Here's how the part is built. I have some questions about the finished solid (model axes, mm). A direction names the side the tool comes from. Coordinates: 2 decimals unless noted, no trailing zeros. Order: outer loops, then holes, each group sorted by start corner. A loop starts at its lowest first (then second) coordinate and runs counter-clockwise, first axis right, second up. Notation, with made-up numbers: (32.25, 6) - (62.25, 6) arc R27 cw to (62.25, 37) - close; hole circle Ø10 at (-35, 65.5). An arc over 180 degrees is marked (long way). Answer in a Markdown table with one row per item. Add a question column.
Item 1: I want a section at D-D (x = 4). Please give me the cut outline in (y, z), plus the area to 3 significant figures.
Item 2: I want a section at A-A (x = -24). Please give me the cut outline in (y, z), plus the area to 3 significant figures.
Item 3: Will these pins go through, and if not, where does the flat tip stop? pin 1 Ø1.5 at (x, z) = (-45.5, 5) entering from -Y; pin 2 Ø1.9 at (y, z) = (40, 4) entering from +X; pin 3 Ø3 at (y, z) = (41.5, 4) entering from -X.
Item 4: If I drill on line 1 along Y through (x, z) = (-56, 3.75); line 2 along Y through (x, z) = (-17, 4.75); line 3 along X through (y, z) = (41, 4), over which ranges is the centre line in solid material (lowest first)? Write a range as from..to.
Item 5: I want a section at C-C (z = 5.25). Please give me the cut outline in (x, y), plus the area to 3 significant figures.
Item 6: Thinking about a two-plate mould opening in Y: for faces 6 (the flat face through (-13, 38.1, 3)), 7 (the flat face through (6.35, 41, 3)), 8 (the flat face through (-43, 69.83, 3)), which applies, +Y half, -Y half, draft (parallel to the pull), parting line (faces both ways), or undercut?
Item 7: I want a section at B-B (y = 67.5). Please give me the cut outline in (x, z) (3 decimals), plus the area to 3 significant figures.
Item 8: On a 3-axis mill with a long thin cutter (end or side, diameter ignored), from which of +Z, -Z, +X, -X, +Y, -Y can I reach the whole of each face in a straight line? I mean faces 1 (the flat face through (-63.45, 59, 3)), 2 (the flat face through (27, 44.45, 3)), 3 (the cylindrical face through (-66.44, 71.28, 3.22)), 4 (the flat face through (-16, 74.13, 3)), 5 (the flat face through (-19.05, 41, 3)). Say none if no direction works.
```python
from build123d import *

# Parameters (mm, degrees)
BOSS_EXTRUDE1_DEPTH = 6.35
SKETCH3_R           = 1.778
SKETCH3_W           = 41
SKETCH3_H           = 21
CUT_EXTRUDE1_DEPTH  = 102.778507746
FILLET1_R           = 10


with BuildPart() as part:
    # Sketch1 → Boss-Extrude1 (new body)
    with BuildSketch(Plane.XY):
        Polygon((19.05, 38.1), (19.05, 44.45), (35.872396717, 44.45), (35.872396717, 74.129883576), (-49.45, 74.129883576), (-69.45, 74.129883576), (-69.45, 44.45), (-44.45, 44.45), (-19.05, 44.45), (-19.05, 38.1), (-6.35, 38.1), (-6.35, 44.45), (6.35, 44.45), (6.35, 38.1), align=None)
    extrude(amount=BOSS_EXTRUDE1_DEPTH)

    # Sketch3 → Cut-Extrude1 (cut, through all)
    with BuildSketch(Plane.XY.offset(6.35)):
        with Locations((-67.4705, 64.289941788)):
            Circle(SKETCH3_R)
        with Locations((-67.4705, 54.289941788)):
            Circle(SKETCH3_R)
        with Locations((-18.4705, 54.289941788)):
            Circle(SKETCH3_R)
        with Locations((-18.4705, 64.289941788)):
            Circle(SKETCH3_R)
        with Locations((-42.95, 59.329883576)):
            Rectangle(SKETCH3_W, SKETCH3_H)
    extrude(amount=-CUT_EXTRUDE1_DEPTH, mode=Mode.SUBTRACT)

    # Fillet1
    fillet1_edges = [part.edges().sort_by_distance(p)[0] for p in [
        (-69.45, 74.129883576, 3.175),
        (35.872396717, 74.129883576, 3.175),
    ]]
    fillet(fillet1_edges, radius=FILLET1_R)


solid = part.part
```
Values follow:
| question | item | result |
|---|---|---|
| 1 | outline | (44.45, 0) - (74.13, 0) - (74.13, 6.35) - (44.45, 6.35) - close |
| 1 | area | 188 mm^2 |
| 2 | outline | (44.45, 0) - (48.83, 0) - (48.83, 6.35) - (44.45, 6.35) - close; (69.83, 0) - (74.13, 0) - (74.13, 6.35) - (69.83, 6.35) - close |
| 2 | area | 55.1 mm^2 |
| 3 | pin 1 | stops at y = 44.45 |
| 3 | pin 2 | stops at x = 19.05 |
| 3 | pin 3 | stops at x = -19.05 |
| 4 | line 1 | y = 44.45..48.83, 69.83..74.13 |
| 4 | line 2 | y = 38.1..53.29, 55.29..63.29, 65.29..74.13 |
| 4 | line 3 | x = -19.05..-6.35, 6.35..19.05 |
| 5 | outline | (-69.45, 44.45) - (-19.05, 44.45) - (-19.05, 38.1) - (-6.35, 38.1) - (-6.35, 44.45) - (6.35, 44.45) - (6.35, 38.1) - (19.05, 38.1) - (19.05, 44.45) - (35.87, 44.45) - (35.87, 64.13) arc R10 ccw to (25.87, 74.13) - (-59.45, 74.13) arc R10 ccw to (-69.45, 64.13) - close; hole circle Ø3.56 at (-67.47, 54.29); hole circle Ø3.56 at (-67.47, 64.29); hole (-63.45, 48.83) - (-22.45, 48.83) - (-22.45, 69.83) - (-63.45, 69.83) - close; hole circle Ø3.56 at (-18.47, 54.29); hole circle Ø3.56 at (-18.47, 64.29) |
| 5 | area | 2,340 mm^2 |
| 6 | face 6 | -Y half |
| 6 | face 7 | draft |
| 6 | face 8 | undercut |
| 7 | outline | (-68.865, 0) - (-63.45, 0) - (-63.45, 6.35) - (-68.865, 6.35) - close; (-22.45, 0) - (35.287, 0) - (35.287, 6.35) - (-22.45, 6.35) - close |
| 7 | area | 401 mm^2 |
| 8 | face 1 | +Z, -Z |
| 8 | face 2 | +Z, -Z, +X, -Y |
| 8 | face 3 | +Z, -Z, -X, +Y |
| 8 | face 4 | +Z, -Z, +X, -X, +Y |
| 8 | face 5 | +Z, -Z, -X, -Y |
